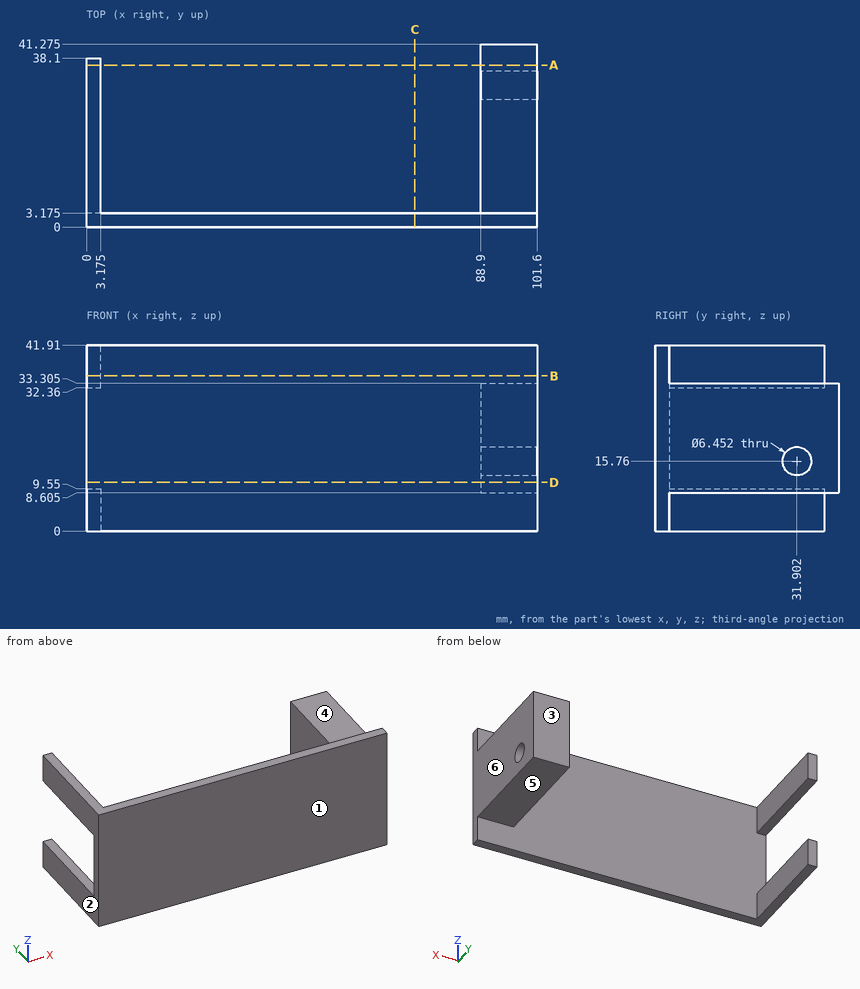
Part print with two shaded views. Sizes in mm from the minimum x, y, z corner. A direction names the side the tool comes from. Coordinates: 2 decimals unless noted, no trailing zeros. Write each loop counter-clockwise with the first axis right and the second up, starting at its lowest first coordinate (ties: lowest second). Pieces come first, ordered by that corner, then holes. Notation, with made-up numbers: (-14, 80) -> (4, 80) arc R15 cw to (4, 100) -> close; hole circle Ø9 at (62, 25). An arc over 180 degrees is marked (long way). Return JSON: item names as keys, results as strings. Group by question number.
Q1. Cut at A-A, the plane y = 36.5. State how many separate pieces and enclosed holes the cut face has, then the cut area to 3 significant figures.
Q2. Pull direction Y, two halves, no side cores. Call the marked faces 1, 2 and 3: released by +Y, released by -Y, zero draft, split by the parting line, or undercut.
Q3. Flat gauge pins, fed straight in: pin 1 (3 mm diameter, centred on y = 25, z = 3.5, fed in from +X) (3 decimals); pin 2 (21 mm diameter, centred on x = 54.5, z = 19.5, fed in from +Y) (3 decimals); pin 3 (1.6 mm diameter, centred on x = 1.5, z = 38, fed in from +Y); pin 4 (6 mm diameter, centred on y = 31.9, z = 15.76, fed in from -X). Where does each tip first touch, or does it go through?
Q4. Cut at D-D, the plane z = 11. Give the cut face in (x, y) (1 decimal).
Q5. Drill centre lines: line 1 (X direction, y = 26, z = 9.5) (1 decimal); line 2 (Y direction, x = 80, z = 29) (1 decimal); line 3 (X direction, y = 16.5, z = 15). Where is each one in solid material? Low to high.
Q6. Cut at C-C, the plane x = 74. Give the cut face in (y, z) (1 decimal).
Q7. Cut at B-B, the plane z = 35. Give the cut face in (x, y) (1 decimal).
Q8. Which spindle directions (+Z, -Z, +X, -X, +Y, -Y) get a long thin tool onto all of the face, cutting with end or side? Do the marked faces 4, 5 and 6. Say none if no direction does.
Returned:
{
 "1": {"separate pieces": "3", "enclosed holes": "0", "area": "374 mm2"},
 "2": {"face 1": "released by -Y", "face 2": "zero draft", "face 3": "released by +Y"},
 "3": {"pin 1": "stops at x = 3.175", "pin 2": "stops at y = 3.175", "pin 3": "stops at y = 38.1", "pin 4": "passes through"},
 "4": {"outline": "(0, 0) -> (101.6, 0) -> (101.6, 41.3) -> (88.9, 41.3) -> (88.9, 3.2) -> (0, 3.2) -> close"},
 "5": {"line 1": "x = 0 to 3.2, 88.9 to 101.6", "line 2": "y = 0 to 3.2", "line 3": "x = 88.9 to 101.6"},
 "6": {"outline": "(0, 0) -> (3.2, 0) -> (3.2, 41.9) -> (0, 41.9) -> close"},
 "7": {"outline": "(0, 0) -> (101.6, 0) -> (101.6, 3.2) -> (3.2, 3.2) -> (3.2, 38.1) -> (0, 38.1) -> close"},
 "8": {"face 4": "+Z, +X, +Y", "face 5": "-Z, +X, +Y", "face 6": "+Z, -Z, +X, +Y, -Y"}
}
